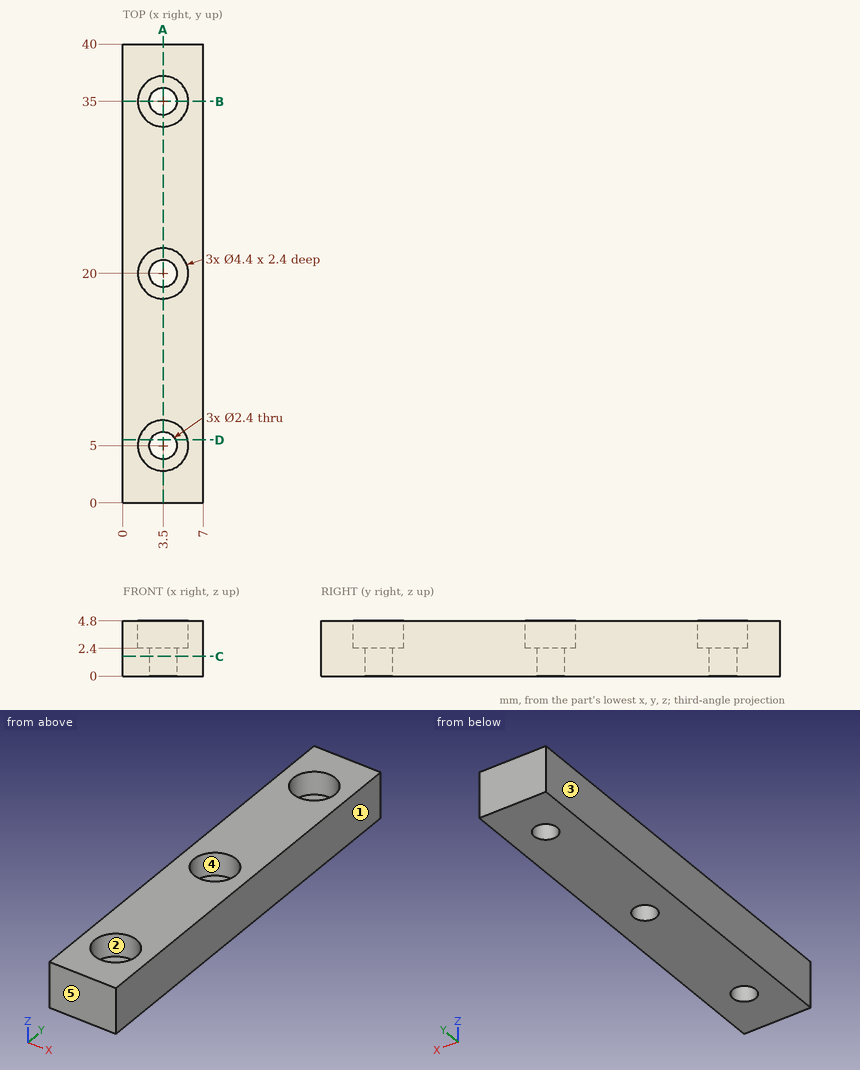
Could you check a few things on this drawing? It's one solid part, dimensions in mm from its lowest x, y, z. A direction names the side the tool comes from. Give positions to 0.01 mm unless a question says otherwise; leave off trailing zeros. Loops run counter-clockwise (first coordinate to the right, second up) from the corner with the lowest first, then second, coordinate; pieces in that order, holes last. Notation, with made-up numbers: (77, 43.5) -> (115, 43.5) arc R7 ccw to (115, 56.5) -> close; hole circle Ø2 at (58.25, -33.75). An arc over 180 degrees is marked (long way). Use one line per item in the form item = value. Start each with the question number.
1) Imagine slicing it at A-A (x = 3.5). Please give me the cut outline in (y, z), then the cut area to 3 significant figures.
2) Imagine slicing it at D-D (y = 5.5). Please give me the cut outline in (x, z).
3) Please list where these lines run through material, in increasing order: line 1 along Y through (x, z) = (3.5, 3.45); line 2 along Y through (x, z) = (1.5, 4.65); line 3 along Z through (x, y) = (5.5, 35.5).
4) Thinking about a two-plate mould opening in Y: for the marked faces 3, 4 and 5, which applies, +Y half, -Y half, draft (parallel to the pull), parting line (faces both ways), or undercut?
5) Which directions (+Z, -Z, +X, -X, +Y, -Y) give clear straight access to the entire face, cutting with the end or side of a thin tool? Please do the marked faces 1 and 2.
6) For P1, Ø3.5, axis at x = 3.5, y = 35, coming from the -Z side; P2, Ø1.3, axis at x = 3.5, y = 21, coming from the +Z side, each with a flat end and sliding along its axis, tell me the tip position at first contact or that it passes through.
7) Imagine slicing it at C-C (z = 1.7). Please give me the cut outline in (x, y).
8) Imagine slicing it at B-B (y = 35). Please give me the cut outline in (x, z).
Check values:
q1.outline = (0, 0) -> (3.8, 0) -> (3.8, 2.4) -> (2.8, 2.4) -> (2.8, 4.8) -> (0, 4.8) -> close; (6.2, 0) -> (18.8, 0) -> (18.8, 2.4) -> (17.8, 2.4) -> (17.8, 4.8) -> (7.2, 4.8) -> (7.2, 2.4) -> (6.2, 2.4) -> close; (21.2, 0) -> (33.8, 0) -> (33.8, 2.4) -> (32.8, 2.4) -> (32.8, 4.8) -> (22.2, 4.8) -> (22.2, 2.4) -> (21.2, 2.4) -> close; (36.2, 0) -> (40, 0) -> (40, 4.8) -> (37.2, 4.8) -> (37.2, 2.4) -> (36.2, 2.4) -> close
q1.area = 143 mm^2
q2.outline = (0, 0) -> (2.41, 0) -> (2.41, 2.4) -> (1.36, 2.4) -> (1.36, 4.8) -> (0, 4.8) -> close; (4.59, 0) -> (7, 0) -> (7, 4.8) -> (5.64, 4.8) -> (5.64, 2.4) -> (4.59, 2.4) -> close
q3.line_1 = 0 to 2.8, 7.2 to 17.8, 22.2 to 32.8, 37.2 to 40
q3.line_2 = 0 to 4.08, 5.92 to 19.08, 20.92 to 34.08, 35.92 to 40
q3.line_3 = 0 to 2.4
q4.face_3 = draft
q4.face_4 = undercut
q4.face_5 = -Y half
q5.face_1 = +Z, -Z, +X, +Y, -Y
q5.face_2 = +Z
q6.P1 = 0
q6.P2 = 2.4
q7.outline = (0, 0) -> (7, 0) -> (7, 40) -> (0, 40) -> close; hole circle Ø2.4 at (3.5, 5); hole circle Ø2.4 at (3.5, 20); hole circle Ø2.4 at (3.5, 35)
q8.outline = (0, 0) -> (2.3, 0) -> (2.3, 2.4) -> (1.3, 2.4) -> (1.3, 4.8) -> (0, 4.8) -> close; (4.7, 0) -> (7, 0) -> (7, 4.8) -> (5.7, 4.8) -> (5.7, 2.4) -> (4.7, 2.4) -> close
